Can you work these out from the model? Positions are in its coordinate system, mm. A direction names the side the tool comes from. Round coordinates to 2 decimals unless told otherwise and drop trailing zeros. Write each loop counter-clockwise with the first axis right and the second up, starting at its lowest first coordinate (ties: lowest second). Pieces come first, ordered by that corner, then holes. Notation, with made-up numbers: (15, 22) -> (30, 22) arc R8 cw to (30, 36) -> close; hole circle Ø4 at (62.25, 13.25). An arc over 180 degrees is marked (long way). Use CSV: the item, a comma, the result in double quotes.
Autodesk Inventor part; units mm, degrees
ref_plane "YZ Plane" through (0, 0, 0) normal (1, 0, 0) x (0, 1, 0)
ref_plane "XZ Plane" through (0, 0, 0) normal (0, 1, 0) x (-1, 0, 0)
ref_plane "XY Plane" through (0, 0, 0) normal (0, 0, 1) x (1, 0, 0)
sketch "Sketch1" plane through (0, 0, 0) normal (0, 1, 0) x (-1, 0, 0)
  line L0 (7.9502, -7.4168) -> (-7.9502, -7.4168)
  line L1 (-7.9502, -7.4168) -> (-7.9502, 7.4168)
  line L2 (-7.9502, 7.4168) -> (7.9502, 7.4168)
  line L3 (7.9502, 7.4168) -> (7.9502, -7.4168)
  point P0 (0, 0)
  point P1 (7.9502, 0)
  point P2 (0, -7.4168)
  dimension "d0" = 14.8336
  dimension "d1" = 15.9004
extrude "Extrusion1" add sketch "Sketch1" along normal mid plane 12.7
sketch "Sketch2" plane through (-7.9502, -6.35, 7.4168) normal (-1, 0, 0) x (0, 0, 1)
  line L0 (0, 0) -> (0, 12.7)
  line L1 (-14.8336, 12.7) -> (0, 12.7)
  line L2 (-14.8336, 0) -> (-14.8336, 12.7)
  line L3 (0, 0) -> (-14.8336, 0)
  line L4 (-13.1318, 12.065) -> (-1.7018, 12.065)
  line L5 (-1.7018, 12.065) -> (-1.7018, 0.635)
  line L6 (-1.7018, 0.635) -> (-13.1318, 0.635)
  line L7 (-13.1318, 0.635) -> (-13.1318, 12.065)
  point P0 (-7.4168, 6.35)
  point P1 (-13.1318, 6.35)
  point P2 (-7.4168, 12.065)
  dimension "d11" = 11.43
  dimension "d12" = 11.43
extrude "Extrusion2" add sketch "Sketch2" along normal blind 11.43 contours L4 L5 L6 L7
sketch "Sketch3" plane through (-19.3802, -6.35, 7.4168) normal (-1, 0, 0) x (0, 0, 1)
  circle A0 centre (-7.4168, 6.35) radius 4.953
  dimension "d10" = 9.906
extrude "Extrusion3" add sketch "Sketch3" along normal blind 11.684
equation "\"d12\" = d11"
properties part number "Plug"
Q1. Suppose I cut it at B-B (y = 0). Write out the boundary of the cut face in (x, z) (3 decimals), and give its area (3 significant figures).
Resolved:
outline,"(-31.064, -4.953) -> (-19.38, -4.953) -> (-19.38, -5.715) -> (-7.95, -5.715) -> (-7.95, -7.417) -> (7.95, -7.417) -> (7.95, 7.417) -> (-7.95, 7.417) -> (-7.95, 5.715) -> (-19.38, 5.715) -> (-19.38, 4.953) -> (-31.064, 4.953) -> close"
area,"482 mm^2"
Q2. On a 3-axis mill with a long thin cutter (end or side, diameter ignored), from which of +Z, -Z, +X, -X, +Y, -Y can I reach the whole of each face in a straight line? I mean faces 1 (the face through (-14, -5.715, 0)), 2 (the face through (-14, 0, -5.715)), 3 (the face through (-19.38, 0.1, -5.2)). Say none if no direction works.
Resolved:
face 1,"+Z, -Z, -X, -Y"
face 2,"-Z, -X, +Y, -Y"
face 3,"-X"
Q3. Please list where these lines run through material, in increasing order: probe 1 along X at (y, z) = (1.5, 6.25); probe 2 along Y at (x, z) = (-8, -2.5) (3 decimals); probe 3 along X at (y, z) = (5, 1.25).
Resolved:
probe 1,"x = -7.95 to 7.95"
probe 2,"y = -5.715 to 5.715"
probe 3,"x = -19.38 to 7.95"
Q4. Suppose I cut it at C-C (x = -16). Write out the boundary of the cut face in (y, z) (3 decimals).
Resolved:
outline,"(-5.715, -5.715) -> (5.715, -5.715) -> (5.715, 5.715) -> (-5.715, 5.715) -> close"
Q5. Suppose I cut it at A-A (z = 0). Write out the boundary of the cut face in (x, y) (3 decimals), and give its area (3 significant figures).
Resolved:
outline,"(-31.064, -4.953) -> (-19.38, -4.953) -> (-19.38, -5.715) -> (-7.95, -5.715) -> (-7.95, -6.35) -> (7.95, -6.35) -> (7.95, 6.35) -> (-7.95, 6.35) -> (-7.95, 5.715) -> (-19.38, 5.715) -> (-19.38, 4.953) -> (-31.064, 4.953) -> close"
area,"448 mm^2"
Q6. Will these pins go through, and if not, where does the flat tip stop? P1, Ø2, axis at x = -20, z = 3.5, coming from the -Y side (3 decimals); P2, Ø5.5, axis at x = -13.5, y = 2, coming from the -Z side (3 decimals); P3, Ø3, axis at x = -23.5, z = 0.5, coming from the +Y side.
Resolved:
P1,"stops at y = -5.715"
P2,"stops at z = -5.715"
P3,"stops at y = 4.95"
Q7. Suppose I cut it at D-D (x = -25). Write out the boundary of the cut face in (y, z).
Resolved:
outline,"circle Ø9.91 at (0, 0)"
